Could you check a few things on this model? Use its own coordinates, in mm. A direction names the side the tool comes from. Give positions to 0.01 mm unless a question says otherwise; leave off trailing zeros. Loops run counter-clockwise (first coordinate to the right, second up) from the corner with the lowest first, then second, coordinate; pieces in that order, holes last. Notation, with made-up numbers: (-24, 33) - (15, 33) arc R32 ccw to (15, 72) - close; hole circle Ø2 at (33.25, 60). An arc over 180 degrees is marked (long way). One line per item, written item: value. Start each with the question number.
Q1. For faces 1 (the face through (-8, 0, 4)), 2 (the face through (-0.5, 8.3, 0)), which set-ups out of +Z, -Z, +X, -X, +Y, -Y let a thin tool reach every point of the face, with its end or its side?
Q2. If we mould it in two halves opening along X, with no side actions, what happens to faces 3 (the face through (0, -7.5, 4)), 4 (the face through (12, 0, 8))? For each: released by +X, released by -X, zero draft, split by the parting line, or undercut.
Q3. I want a section at C-C (z = 4). Please give me the cut outline in (x, y).
Q4. I'm going to push flat-ended pins straight in: P1, Ø1.5, axis at x = 10.5, z = 2, coming from the +Y side; P2, Ø2.5, axis at y = 1.5, z = 2, coming from the +X side; P3, Ø4, axis at x = 2.5, z = 4, coming from the +Y side. Where does each tip first touch, or does it pass through?
Q5. If I drill on line 1 (Y direction, x = 21.5, z = 2.75); line 2 (X direction, y = 17, z = 1.75); line 3 (Y direction, x = 30, z = 1.75), over which ranges is the centre line in solid material (lowest first)? Write a range as from..to.
```python
from build123d import *

# Parameters (mm, degrees)
F0_R     = 35
F0_W     = 15.5
F0_H     = 15.5
F1_DEPTH = 8
F2_R     = 7.99999


# Not quite as in the source:
# - a fillet or chamfer is up to 0.001 mm smaller than in the source, because OpenCascade refuses the exact size


with BuildPart() as f1:
    # F0 (on Top) → F1 (new body)
    with BuildSketch(Plane.XY):
        Circle(F0_R)
        with Locations((-0.25, 0.25)):
            Rectangle(F0_W, F0_H, mode=Mode.SUBTRACT)
    extrude(amount=F1_DEPTH)

    # F2 (radius 8 in the source; OpenCascade refuses exactly that, so slightly less here)
    f2_edges = [f1.edges().sort_by_distance(p)[0] for p in [
        (-35, 0, 8),
    ]]
    fillet(f2_edges, radius=F2_R)


solid = f1.part
```
Worked answers:
1. face 1: +Z, -Z
1. face 2: -Z, +X, -X, +Y, -Y
2. face 3: undercut
2. face 4: zero draft
3. outline: circle Ø67.86 at (0, 0); hole (-8, -7.5) - (7.5, -7.5) - (7.5, 8) - (-8, 8) - close
4. P1: stops at y = 33.41
4. P2: stops at x = 34.94
4. P3: stops at y = 34.67
5. line 1: y = -27..27
5. line 2: x = -30.37..30.37
5. line 3: y = -17.65..17.65
